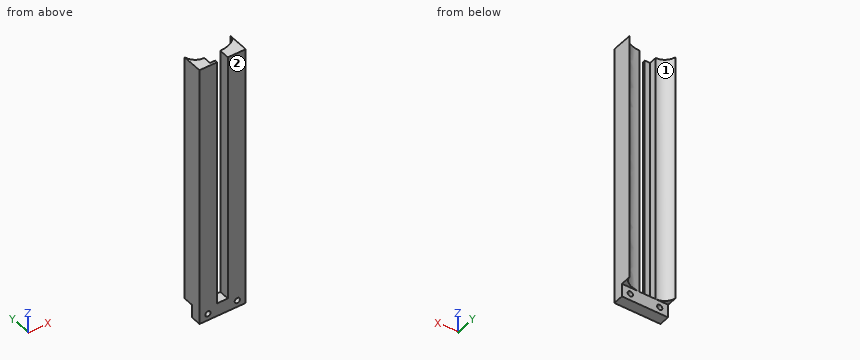
```python
from build123d import *

# Parameters (mm, degrees)
SKETCH1_W           = 27.94
SKETCH1_H           = 6.35
BOSS_EXTRUDE1_DEPTH = 7.9502
SKETCH2_W           = 10.795
SKETCH2_H           = 6.35
BOSS_EXTRUDE2_DEPTH = 151.60625
SKETCH4_R           = 1.5875
CUT_EXTRUDE1_DEPTH  = 161.292682729
BOSS_EXTRUDE3_DEPTH = 151.60625


with BuildPart() as part:
    # Sketch1 → Boss-Extrude1 (new body)
    with BuildSketch(Plane.XY):
        Rectangle(SKETCH1_W, SKETCH1_H)
    extrude(amount=BOSS_EXTRUDE1_DEPTH)

    # Sketch2 → Boss-Extrude2 (add)
    with BuildSketch(Plane.XY.offset(7.9502)):
        Polygon((-3.302, -3.175), (-3.302, -1.5875), (-6.477, -1.5875), (-6.477, 3.175), (-13.97, 3.175), (-13.97, -3.175), align=None)
        with Locations((8.5725, 0)):
            Rectangle(SKETCH2_W, SKETCH2_H)
    extrude(amount=BOSS_EXTRUDE2_DEPTH)

    # Sketch4 → Cut-Extrude1 (cut, through all)
    with BuildSketch(Plane(origin=(0, 3.175, 0), x_dir=(1, 0, 0), z_dir=(0, 1, 0))):
        with Locations(Location((-8.89, -3.9751, 0), (0, 0, 270))):
            Circle(SKETCH4_R)
        with Locations(Location((8.89, -3.9751, 0), (0, 0, 270))):
            Circle(SKETCH4_R)
    extrude(amount=-CUT_EXTRUDE1_DEPTH, mode=Mode.SUBTRACT)

    # Sketch5 → Boss-Extrude3 (add)
    with BuildSketch(Plane.XY.offset(159.55645)):
        with BuildLine():
            Line((-13.97, 3.175), (-13.97, 9.525))
            ThreePointArc((-13.97, 9.525), (-11.38789475, 4.976014194), (-6.477, 3.175))
            Line((-6.477, 3.175), (-13.97, 3.175))
        make_face()
        with BuildLine():
            Line((3.175, 3.175), (13.97, 3.175))
            Line((13.97, 3.175), (13.97, 9.525))
            add(Edge.make_bspline(
                [(3.175, 3.175), (13.97, 3.175), (13.97, 9.525)],
                knots=[4.71238898, 4.71238898, 4.71238898, 6.283185307, 6.283185307, 6.283185307], degree=2, weights=[1, 0.707106781, 1]))
        make_face()
    extrude(amount=-BOSS_EXTRUDE3_DEPTH)


solid = part.part
```
Source: CAD feature listing. Evaluate the final solid. Frame: model axes, mm. Face numbers are marked on the shaded views. A direction names the side the tool comes from. Give positions to 0.01 mm unless a question says otherwise; leave off trailing zeros. Write each loop counter-clockwise with the first axis right and the second up, starting at its lowest first coordinate (ties: lowest second). Pieces come first, ordered by that corner, then holes. Notation, with made-up numbers: (70.25, 9.5) - (86.25, 9.5) arc R15 cw to (86.25, 18.5) - close; hole circle Ø6 at (65, 84.25). An arc over 180 degrees is marked (long way). One line per item, written item: value. Start each with the question number.
Q1. Section query A-A, the plane y = 1. Return the cut outline in (x, z) (1 decimal).
Q2. Material intervals for probe 1 along X at (y, z) = (0.25, 105) (3 decimals); probe 2 along Z at (x, y) = (-9.5, -1); probe 3 along X at (y, z) = (6, 67.5), sorted ascending. Write a range as from..to.
Q3. First-contact query: pin 1 Ø5 at (x, y) = (10, 7) entering from -Z; pin 2 Ø1.6 at (x, z) = (-5, 49) entering from +Y; pin 3 Ø5 at (x, z) = (8.89, 3.98) entering from +Y (3 decimals). Flat tips, straight axial feed; report the tip coordinate or a pass-through.
Q4. Set-up query: the marked faces 1 and 2. Return all of +Z, -Z, +X, -X, +Y, -Y with unobstructed straight access to the full face (end or side cutting, diameter ignored); none if empty.
Q5. Section query B-B, the plane x = -8.89. Return the cut outline in (y, z) (3 decimals), then the cut area to 3 significant figures.
Answer:
1. outline: (-14, 0) - (14, 0) - (14, 159.6) - (3.2, 159.6) - (3.2, 8) - (-6.5, 8) - (-6.5, 159.6) - (-14, 159.6) - close; hole circle Ø3.2 at (-8.9, 4); hole circle Ø3.2 at (8.9, 4)
2. probe 1: x = -13.97..-6.477, 3.175..13.97
2. probe 2: z = 0..2.51, 5.44..159.56
2. probe 3: x = -13.97..-12.39, 12.15..13.97
3. pin 1: stops at z = 7.95
3. pin 2: stops at y = -1.59
3. pin 3: stops at y = 3.175
4. face 1: +Z, -Z, +Y
4. face 2: +Z, -Z, +X, -X, -Y
5. outline: (-3.175, 0) - (3.175, 0) - (3.175, 2.388) - (-3.175, 2.388) - close; (-3.175, 5.563) - (3.175, 5.563) - (3.175, 7.95) - (3.568, 7.95) - (3.568, 159.556) - (-3.175, 159.556) - close
5. area: 1,050 mm2
